Autodesk Inventor part; units mm, degrees
ref_plane "YZ Plane" through (0, 0, 0) normal (1, 0, 0) x (0, 1, 0)
ref_plane "XZ Plane" through (0, 0, 0) normal (0, 1, 0) x (-1, 0, 0)
ref_plane "XY Plane" through (0, 0, 0) normal (0, 0, 1) x (1, 0, 0)
sketch "Sketch1" plane through (0, 0, 0) normal (0, 0, 1) x (1, 0, 0)
  line L0 (-6.2, 0) -> (37.2, 0) construction
  line L1 (0, -7.2) -> (0, 8.2) construction
  line L2 (1.5, 0) -> (19, 0)
  line L3 (1.5, 0) -> (1.5, 1.5)
  line L4 (19, 0) -> (19, 3)
  line L5 (17, 5) -> (14, 5)
  line L6 (10.5, 1.5) -> (1.5, 1.5)
  line L7 (10.5, 1.5) -> (14, 5)
  line L8 (10.5, 1.5) -> (15.4497, 1.5) construction
  arc A0 (19, 3) -> (17, 5) centre (17, 3) ccw
  line L9 (19, 3) -> (31, 3)
  line L10 (31, 3) -> (31, -5)
  line L11 (31, -5) -> (0, -5)
  line L12 (1.5, 6) -> (0, 6)
  line L13 (0, 6) -> (0, -5)
  line L14 (1.5, 1.5) -> (1.5, 6)
  point P0 (0, 0)
  point P1 (19, 5)
  dimension "d1" = 19
  dimension "d2" = 1.5
  dimension "d3" = 1.5
  dimension "d4" = 5
  dimension "d6" = 45
  dimension "d7" = 10.5
  dimension "d8" = 2
  dimension "d9" = 12
  dimension "d10" = 5
  dimension "d18" = 6
revolve "Revolution1" add sketch "Sketch1" angle 360 about axis through (0, -10, 0) along (0, 1, 0) contours L2 L4 L9 L10 L11 L13 L12 L14 L3
sketch "Sketch2" plane through (0, -5, 0) normal (0, -1, 0) x (1, 0, 0)
  circle A0 centre (0, 0) radius 31 construction
  circle A1 centre (0, 0) radius 19 construction
  circle A2 centre (0, 0) radius 19 construction
  line L0 (0, 19) -> (0, 31) construction
  circle A3 centre (0, 0) radius 31 construction
  circle A4 centre (0, 25) radius 3.25
  dimension "d12" = 6.5
extrude "Extrusion1" cut sketch "Sketch2" against normal up to surface (8 mm away)
pattern_circular "Circular Pattern1" count 6 over 360 about axis through (0, -1, 0) along (0, -1, 0) of "Extrusion1"
properties part number "MouldBase"
Input: part model. Units: mm. Frame: model coordinates. A direction names the side the tool comes from. Give positions to 0.01 mm unless a question says otherwise; leave off trailing zeros. Order: outer loops, then holes, each group sorted by start corner. A loop starts at its lowest first (then second) coordinate and runs counter-clockwise, first axis right, second up.
1. Pin query (flat end, axial travel): pin 1 Ø3 at (y, z) = (-0.5, 13.5) entering from +X; pin 2 Ø4 at (y, z) = (-2.5, 16) entering from +X; pin 3 Ø3 at (y, z) = (-2, -11) entering from +X. Return the tip coordinate at first contact, or that it passes through.
Computed:
pin 1: stops at x = 28.58
pin 2: stops at x = 27.66
pin 3: stops at x = 29.51
2. Cut plane B-B (y = -1.25). Return loops of the section in (x, z), and give its area (3 significant figures).
Computed:
outline: circle Ø62 at (0, 0); hole circle Ø6.5 at (-21.65, -12.5); hole circle Ø6.5 at (-21.65, 12.5); hole circle Ø6.5 at (0, -25); hole circle Ø6.5 at (0, 25); hole circle Ø6.5 at (21.65, -12.5); hole circle Ø6.5 at (21.65, 12.5)
area: 2,820 mm2
3. Set-up query: faces 1 (the face through (8.767, 1.521, 16.856)), 2 (the face through (20.946, -1.056, -15.673)). Return all of +Z, -Z, +X, -X, +Y, -Y with unobstructed straight access to the full face (end or side cutting, diameter ignored); none if empty.
Computed:
face 1: +Y
face 2: +Y, -Y
4. Cut plane C-C (z = -23). Return loops of the section in (x, y).
Computed:
outline: (-20.78, -5) - (-2.56, -5) - (-2.56, 3) - (-20.78, 3) - close; (2.56, -5) - (20.78, -5) - (20.78, 3) - (2.56, 3) - close
5. Draft query along X for faces 3 (the face through (-18.55, -1.06, -11.52)), 4 (the face through (0, 6, 0)), 5 (the face through (-4.036, -1.056, 30.736)). Return one class per face: released by +X, released by -X, zero draft, split by the parting line, or undercut.
Computed:
face 3: undercut
face 4: zero draft
face 5: split by the parting line
6. Cut plane D-D (z = -12.5). Return loops of the section in (x, y).
Computed:
outline: (-28.37, -5) - (-24.9, -5) - (-24.9, 3) - (-28.37, 3) - close; (-18.4, -5) - (18.4, -5) - (18.4, 3) - (14.31, 3) - (14.31, 0) - (-14.31, 0) - (-14.31, 3) - (-18.4, 3) - close; (24.9, -5) - (28.37, -5) - (28.37, 3) - (24.9, 3) - close
7. Cut plane A-A (x = 0). Return loops of the section in (y, z).
Computed:
outline: (-5, -31) - (3, -31) - (3, -28.25) - (-5, -28.25) - close; (-5, -21.75) - (3, -21.75) - (3, -19) - (0, -19) - (0, -1.5) - (6, -1.5) - (6, 1.5) - (0, 1.5) - (0, 19) - (3, 19) - (3, 21.75) - (-5, 21.75) - close; (-5, 28.25) - (3, 28.25) - (3, 31) - (-5, 31) - close
8. Line query: probe 1 along X at (y, z) = (2.05, 0); probe 2 along Z at (x, y) = (0, 1.95); probe 3 along Z at (x, y) = (0, -2). Output: solid intervals per line, ascending.
Computed:
probe 1: x = -31 to -19, -1.5 to 1.5, 19 to 31
probe 2: z = -31 to -28.25, -21.75 to -19, -1.5 to 1.5, 19 to 21.75, 28.25 to 31
probe 3: z = -31 to -28.25, -21.75 to 21.75, 28.25 to 31
